```python
from build123d import *

# Parameters (mm, degrees)
SKETCH_5_W               = 4
SKETCH_5_H               = 2
EXTRUDE_1_DEPTH          = 22
SKETCH_6_W               = 3.5
SKETCH_6_H               = 6.2
EXTRUDE_2_DEPTH          = 1.2
CUT_EXTRUDE_1_REACH      = 62.614
CUT_EXTRUDE_1_END_RADIUS = 28.5
SKETCH_7_R               = 1.4


with BuildPart() as part:
    # 草图4 → 旋转1 (revolve)
    with BuildSketch(Plane(origin=(0, 0, 0), x_dir=(0, 0, -1), z_dir=(1, 0, 0))):
        with BuildLine():
            Line((16.5, 43.2), (16.5, 42))
            Line((16.5, 42), (22, 42))
            ThreePointArc((22, 42), (25.535533906, 40.535533906), (27, 37))
            Line((27, 37), (27, 0))
            Line((27, 0), (28.5, 0))
            Line((28.5, 0), (28.5, 38.27179677))
            ThreePointArc((28.5, 38.27179677), (26.082575695, 43.563299392), (20.5, 45.2))
            Line((20.5, 45.2), (20.5, 43.2))
            Line((20.5, 43.2), (16.5, 43.2))
        make_face()
    revolve(axis=Axis((0, 0, 0), (0, 1, 0)))

    # 草图5 → 凸台-拉伸1 (add)
    with BuildSketch(Plane.XZ):
        with Locations((26, 2.1)):
            Rectangle(SKETCH_5_W, SKETCH_5_H)
        with Locations((26, -2.1)):
            Rectangle(SKETCH_5_W, SKETCH_5_H)
        Polygon((16.684678752, -22.698711306), (14.684678752, -19.234609691), (12.952627944, -20.234609691), (14.952627944, -23.698711306), align=None)
        Polygon((13.047372056, -24.798711306), (11.315321248, -25.798711306), (9.315321248, -22.334609691), (11.047372056, -21.334609691), align=None)
        Polygon((-11.315321248, -25.798711306), (-9.315321248, -22.334609691), (-11.047372056, -21.334609691), (-13.047372056, -24.798711306), align=None)
        Polygon((-14.952627944, -23.698711306), (-16.684678752, -22.698711306), (-14.684678752, -19.234609691), (-12.952627944, -20.234609691), align=None)
        with Locations((-26, -2.1)):
            Rectangle(SKETCH_5_W, SKETCH_5_H)
        with Locations((-26, 2.1)):
            Rectangle(SKETCH_5_W, SKETCH_5_H)
        Polygon((-16.684678752, 22.698711306), (-14.684678752, 19.234609691), (-12.952627944, 20.234609691), (-14.952627944, 23.698711306), align=None)
        Polygon((-13.047372056, 24.798711306), (-11.315321248, 25.798711306), (-9.315321248, 22.334609691), (-11.047372056, 21.334609691), align=None)
        Polygon((11.315321248, 25.798711306), (9.315321248, 22.334609691), (11.047372056, 21.334609691), (13.047372056, 24.798711306), align=None)
        Polygon((14.952627944, 23.698711306), (16.684678752, 22.698711306), (14.684678752, 19.234609691), (12.952627944, 20.234609691), align=None)
    extrude(amount=-EXTRUDE_1_DEPTH)

    # 草图6 → 凸台-拉伸2 (add)
    with BuildSketch(Plane(origin=(0, 22, 0), x_dir=(1, 0, 0), z_dir=(0, 1, 0))):
        Polygon((9.315321248, -22.334609691), (11.065321248, -25.365698604), (16.434678752, -22.265698604), (14.684678752, -19.234609691), align=None)
        with Locations((25.75, 0)):
            Rectangle(SKETCH_6_W, SKETCH_6_H)
        Polygon((-14.684678752, -19.234609691), (-16.434678752, -22.265698604), (-11.065321248, -25.365698604), (-9.315321248, -22.334609691), align=None)
        with Locations((-25.75, 0)):
            Rectangle(SKETCH_6_W, SKETCH_6_H)
        Polygon((-9.315321248, 22.334609691), (-11.065321248, 25.365698604), (-16.434678752, 22.265698604), (-14.684678752, 19.234609691), align=None)
        Polygon((14.684678752, 19.234609691), (16.434678752, 22.265698604), (11.065321248, 25.365698604), (9.315321248, 22.334609691), align=None)
    extrude(amount=-EXTRUDE_2_DEPTH)

    # 切除-拉伸1: up to this cylinder (the profile starts inside it)
    cut_extrude_1_end = Plane(origin=(0, 12.2, 0), z_dir=(0, -1, 0)) * Cylinder(CUT_EXTRUDE_1_END_RADIUS, 183.228, mode=Mode.PRIVATE)
    # 草图7 → 切除-拉伸1 (cut, up to the surface)
    with BuildSketch(Plane.XY, mode=Mode.PRIVATE) as cut_extrude_1_sk1:
        with Locations((0, 12.2)):
            Circle(SKETCH_7_R)
    cut_extrude_1_tool1 = extrude(cut_extrude_1_sk1.sketch, amount=-CUT_EXTRUDE_1_REACH, mode=Mode.PRIVATE) & cut_extrude_1_end
    add(cut_extrude_1_tool1.solids().sort_by_distance((0, 12.2, 0))[0], mode=Mode.SUBTRACT)


solid = part.part
```
For this review, take the finished solid that the model builds, in its own axes (mm). A direction names the side the tool comes from. Give positions to 0.01 mm unless a question says otherwise; leave off trailing zeros. Write each loop counter-clockwise with the first axis right and the second up, starting at its lowest first coordinate (ties: lowest second). Pieces come first, ordered by that corner, then holes. Notation, with made-up numbers: M 0.5,45.25 L 14.5,45.25 A14 cw 14.5,68.25 Z; hole C 12.5,89.25 d8. An arc over 180 degrees is marked long. One line per item, written item: value.
1) Take a section at B-B, the plane z = 0. Write out the cut boundary in (x, y), then the cut area to 3 significant figures.
Results are:
outline: M -28.5,0 L -27,0 L -27,20.8 L -24,20.8 L -24,22 L -27,22 L -27,37 A5 cw -22,42 L -16.5,42 L -16.5,43.2 L -20.5,43.2 L -20.5,45.2 A7 ccw -28.5,38.27 Z; M 16.5,42 L 22,42 A5 cw 27,37 L 27,22 L 24,22 L 24,20.8 L 27,20.8 L 27,0 L 28.5,0 L 28.5,38.27 A7 ccw 20.5,45.2 L 20.5,43.2 L 16.5,43.2 Z
area: 185 mm²
2) For line 1 (X direction, y = 12, z = 23.5); line 2 (X direction, y = 18, z = 0), list the stretches that pass through material, from the lowest coordinate up. Write a range as from..to.
Results are:
line 1: x = -16.12..-13.29, -12.3..-9.99, 9.99..12.3, 13.29..16.12
line 2: x = -28.5..-27, 27..28.5
3) For faces 1 (the cylindrical face through (6.32, 42.59, -15.24)), 2 (the cylindrical face through (20.013, 44.186, 4.444)), 3 (the flat face through (25, 10, 1.1)), list the 3-axis set-ups (+Z, -Z, +X, -X, +Y, -Y) from which the entire face can be reached by the end or side of a thin tool; tool diameter is ignored.
Results are:
face 1: +Y, -Y
face 2: +Y
face 3: -Y
4) For P1, Ø10, axis at x = 10, z = -8.5, coming from the +Y side; P2, Ø3.5, axis at x = 25, z = 0, coming from the +Y side; P3, Ø0.7, axis at x = 26, z = -0.5, coming from the -Y side, all flat-tipped, find the tip position at first contact; note any pin that passes through.
Results are:
P1: stops at y = 43.2
P2: stops at y = 45.05
P3: stops at y = 20.8
5) Take a section at A-A, the plane x = 0. Write out the cut boundary in (y, z), then the cut area to 3 significant figures.
Results are:
outline: M 0,-28.5 L 10.8,-28.5 L 10.8,-27 L 0,-27 Z; M 0,27 L 37,27 A5 cw 42,22 L 42,16.5 L 43.2,16.5 L 43.2,20.5 L 45.2,20.5 A7 ccw 38.27,28.5 L 0,28.5 Z; M 13.6,-28.5 L 38.27,-28.5 A7 ccw 45.2,-20.5 L 43.2,-20.5 L 43.2,-16.5 L 42,-16.5 L 42,-22 A5 cw 37,-27 L 13.6,-27 Z
area: 173 mm²
6) The part is to be moulded in two halves that separate along Z. For faces 4 (the flat face through (25, 0, -2)), 5 (the flat face through (-10.03, 10.85, 23.57)), say which applies: +Z half, -Z half, draft (parallel to the pull), parting line (faces both ways), or undercut.
Results are:
face 4: draft
face 5: undercut
